```python
from build123d import *

# Parameters (mm, degrees)
F0_R     = 4
F1_DEPTH = 3


with BuildPart() as f1:
    # F0 (on Front) → F1 (new body)
    with BuildSketch(Plane.XZ):
        with BuildLine():
            ThreePointArc((-42.428788, 22.197763), (-22.393428, 40.636528), (0.736568, 26.269656))
            Line((0.736568, 26.269656), (7.82161, 7.734496))
            Line((7.82161, 7.734496), (445.831745, 440.866256))
            Line((445.831745, 440.866256), (409.571118, 551.809463))
            ThreePointArc((409.571118, 551.809463), (403.393924, 553.012383), (397.791506, 555.879027))
            Line((397.791506, 555.879027), (-153.711431, 555.879027))
            Line((-153.711431, 555.879027), (-163.711431, 555.879027))
            Line((-163.711431, 555.879027), (-176.433934, 530.299822))
            Line((-176.433934, 530.299822), (-292.672837, 296.595913))
            Line((-292.672837, 296.595913), (-429.805557, 108.635613))
            ThreePointArc((-429.805557, 108.635613), (-433.055197, 105.145969), (-437.038546, 102.524765))
            Line((-437.038546, 102.524765), (-467.979575, 87.098137))
            ThreePointArc((-467.979575, 87.098137), (-479.031049, 77.063624), (-483.216559, 62.73505))
            Line((-483.216559, 62.73505), (-444.218322, 62.364245))
            ThreePointArc((-444.218322, 62.364245), (-439.992581, 60.566627), (-438.27564, 56.307469))
            ThreePointArc((-438.27564, 56.307469), (-440.073258, 52.081729), (-444.332415, 50.364787))
            Line((-444.332415, 50.364787), (-483.330653, 50.735592))
            Line((-483.330653, 50.735592), (-473.742625, 39.200006))
            ThreePointArc((-473.742625, 39.200006), (-462.016917, 29.862605), (-447.542263, 25.968544))
            Line((-447.542263, 25.968544), (-119.640526, 6.942116))
            ThreePointArc((-119.640526, 6.942116), (-120.273154, 17.038104), (-119.882564, 27.146349))
            ThreePointArc((-119.882564, 27.146349), (-118.168468, 30.486744), (-114.612815, 31.692435))
            Line((-114.612815, 31.692435), (-99.287074, 30.803162))
            ThreePointArc((-99.287074, 30.803162), (-100.086144, 23.806602), (-100.266839, 16.766878))
            ThreePointArc((-100.266839, 16.766878), (-99.974524, 11.247746), (-99.30184, 5.761968))
            Line((-99.30184, 5.761968), (-45.922757, 2.664658))
            Line((-45.922757, 2.664658), (-42.428788, 22.197763))
        make_face()
        with BuildLine():
            ThreePointArc((-219.185589, 82.205842), (-234.185589, 97.205842), (-219.185589, 112.205842))
            Line((-219.185589, 112.205842), (-139.185589, 112.205842))
            ThreePointArc((-139.185589, 112.205842), (-124.185589, 97.205842), (-139.185589, 82.205842))
            Line((-139.185589, 82.205842), (-219.185589, 82.205842))
        make_face(mode=Mode.SUBTRACT)
        with BuildLine():
            ThreePointArc((-238.884885, 257.620199), (-269.539195, 249.087128), (-278.072266, 279.741438))
            Line((-278.072266, 279.741438), (-223.998126, 375.532812))
            ThreePointArc((-223.998126, 375.532812), (-193.343817, 384.065883), (-184.810746, 353.411573))
            Line((-184.810746, 353.411573), (-238.884885, 257.620199))
        make_face(mode=Mode.SUBTRACT)
        with Locations((-83.001788, 494.079027)):
            Circle(F0_R, mode=Mode.SUBTRACT)
        with Locations((9.507399, 72.687717)):
            Circle(F0_R, mode=Mode.SUBTRACT)
        with Locations((386.357424, 494.079027)):
            Circle(F0_R, mode=Mode.SUBTRACT)
        with BuildLine():
            ThreePointArc((-114.612815, 31.692435), (-104.514185, 27.041692), (-100.266839, 16.766878))
            ThreePointArc((-100.266839, 16.766878), (-100.086144, 23.806602), (-99.287074, 30.803162))
            Line((-99.287074, 30.803162), (-114.612815, 31.692435))
        make_face()
        with BuildLine():
            Line((-153.711431, 555.879027), (397.791506, 555.879027))
            ThreePointArc((397.791506, 555.879027), (388.241023, 574.279027), (397.791506, 592.679027))
            Line((397.791506, 592.679027), (-153.711431, 592.679027))
            ThreePointArc((-153.711431, 592.679027), (-135.311431, 574.279027), (-153.711431, 555.879027))
        make_face()
        with BuildLine():
            Line((-153.711431, 592.679027), (397.791506, 592.679027))
            ThreePointArc((397.791506, 592.679027), (403.393924, 595.545671), (409.571118, 596.748591))
            Line((409.571118, 596.748591), (418.046209, 622.679027))
            Line((418.046209, 622.679027), (406.046209, 622.679027))
            ThreePointArc((406.046209, 622.679027), (403.924889, 623.557707), (403.046209, 625.679027))
            ThreePointArc((403.046209, 625.679027), (403.924889, 627.800347), (406.046209, 628.679027))
            Line((406.046209, 628.679027), (420.007247, 628.679027))
            Line((420.007247, 628.679027), (445.831745, 707.691799))
            Line((445.831745, 707.691799), (7.82161, 1140.823559))
            Line((7.82161, 1140.823559), (0.736568, 1122.288398))
            ThreePointArc((0.736568, 1122.288398), (-22.393428, 1107.921526), (-42.428788, 1126.360291))
            Line((-42.428788, 1126.360291), (-45.922757, 1145.893396))
            Line((-45.922757, 1145.893396), (-447.542263, 1122.58951))
            ThreePointArc((-447.542263, 1122.58951), (-462.016917, 1118.695449), (-473.742625, 1109.358048))
            Line((-473.742625, 1109.358048), (-483.330653, 1097.822462))
            Line((-483.330653, 1097.822462), (-444.332415, 1098.193267))
            ThreePointArc((-444.332415, 1098.193267), (-440.073258, 1096.476326), (-438.27564, 1092.250585))
            ThreePointArc((-438.27564, 1092.250585), (-439.992581, 1087.991428), (-444.218322, 1086.19381))
            Line((-444.218322, 1086.19381), (-483.216559, 1085.823005))
            ThreePointArc((-483.216559, 1085.823005), (-479.031049, 1071.494431), (-467.979575, 1061.459917))
            Line((-467.979575, 1061.459917), (-437.038546, 1046.033289))
            ThreePointArc((-437.038546, 1046.033289), (-433.055197, 1043.412085), (-429.805557, 1039.922441))
            Line((-429.805557, 1039.922441), (-292.672837, 851.962142))
            Line((-292.672837, 851.962142), (-178.632735, 622.679027))
            Line((-178.632735, 622.679027), (-176.433934, 618.258232))
            Line((-176.433934, 618.258232), (-163.711431, 592.679027))
            Line((-163.711431, 592.679027), (-153.711431, 592.679027))
        make_face()
        with Locations((-83.001788, 654.479027)):
            Circle(F0_R, mode=Mode.SUBTRACT)
        with BuildLine():
            ThreePointArc((-281.759139, 875.347847), (-276.070425, 895.784053), (-255.634219, 890.095339))
            Line((-255.634219, 890.095339), (-194.186333, 781.241505))
            ThreePointArc((-194.186333, 781.241505), (-199.875047, 760.805298), (-220.311253, 766.494012))
            Line((-220.311253, 766.494012), (-281.759139, 875.347847))
        make_face(mode=Mode.SUBTRACT)
        with Locations((386.357424, 654.479027)):
            Circle(F0_R, mode=Mode.SUBTRACT)
        with Locations((9.507399, 1075.870338)):
            Circle(F0_R, mode=Mode.SUBTRACT)
    extrude(amount=F1_DEPTH)


solid = f1.part
```
Geometry check sheet. Reference: the model listing, model coordinates, mm. A direction names the side the tool comes from. Give positions to 0.01 mm unless a question says otherwise; leave off trailing zeros. Order: outer loops, then holes, each group sorted by start corner. A loop starts at its lowest first (then second) coordinate and runs counter-clockwise, first axis right, second up. Notation, with made-up numbers: (22.5, 83) -> (43.5, 83) arc R37 ccw to (43.5, 122) -> close; hole circle Ø11 at (-4.5, 4.5). An arc over 180 degrees is marked (long way). Write each question's results on one line, items separated by ' | '. Start each with the question number.
(1) Gauge pin test, flat ends, axial feed: P1, Ø1.5, axis at y = -0.5, z = 1019.5, coming from the +X side; P2, Ø1.5, axis at x = 414, y = -1.5, coming from the -Z side; P3, Ø0.9, axis at x = -160.5, y = -2, coming from the -Z side. Record the tip position at first contact, or that the pin passes through.
(2) Sectioned sample at B-B (y = -1.5). Give the number of separate pieces and of enclosed holes in the cut face, plus the area to 3 significant figures.
(3) Mould release check, pull along Z, two halves, no side actions. Record for faces 1 (the face through (-243.921, -1.479, 1134.405)), 2 (the face through (-25, 0, 582)), 3 (the face through (-276.356, -1.479, 895.619)): pulls with the +Z half, pulls with the -Z half, needs draft (parallel to the pull), parting line crosses it, or undercut.
(4) Scan lines: line 1 (Z direction, x = -231, y = -1.9); line 2 (Z direction, x = -195.5, y = -0.7); line 3 (X direction, y = -1, z = 349.5). Record each from-to range of solid material in increasing order.
(5) Access from +Z, -Z, +X, -X, +Y, -Y to the whole of each face (thin tool, end or side, straight path). Record for faces 4 (the face through (-225.34, -1.48, 836.43)), 5 (the face through (427.955, -1.479, 495.561)), 6 (the face through (-360.3, -1.5, 203.9)).
(6) Sectioned sample at D-D (x = 171). Enter the section's corners in (y, z).
(7) Sectioned sample at C-C (z = 967). Enter the section's corners in (x, y).
(8) Sectioned sample at A-A (z = 337.5). Enter the section's corners in (x, y), plus the area to 3 significant figures.
Answer below:
1) P1: x = 131.27 | P2: z = 408.65 | P3: z = 9.29
2) separate pieces: 1 | enclosed holes: 9 | area: 638,000 mm2
3) face 1: pulls with the +Z half | face 2: needs draft | face 3: undercut
4) line 1: 13.4 to 87.96, 106.45 to 271.59, 363.13 to 420.59, 727.97 to 785.43, 846.46 to 1135.15 | line 2: 11.34 to 82.21, 112.21 to 334.48, 385.14 to 491.97, 656.59 to 764.54, 783.57 to 1137.21 | line 3: -266.36 to -238.69, -187.02 to 353.44
5) face 4: +Y, -Y | face 5: +X, +Y, -Y | face 6: -X, +Y, -Y
6) outline: (-3, 169.1) -> (0, 169.1) -> (0, 979.46) -> (-3, 979.46) -> close
7) outline: (-376.6, -3) -> (183.6, -3) -> (183.6, 0) -> (-376.6, 0) -> close
8) outline: (-272.33, -3) -> (-245.47, -3) -> (-245.47, 0) -> (-272.33, 0) -> close; (-193.79, -3) -> (341.3, -3) -> (341.3, 0) -> (-193.79, 0) -> close | area: 1,690 mm2
